The model under review builds one solid part; all positions refer to its coordinate system, in mm. Round coordinates to 2 decimals unless told otherwise and drop trailing zeros. Order: outer loops, then holes, each group sorted by start corner. A loop starts at its lowest first (then second) coordinate and runs counter-clockwise, first axis right, second up.
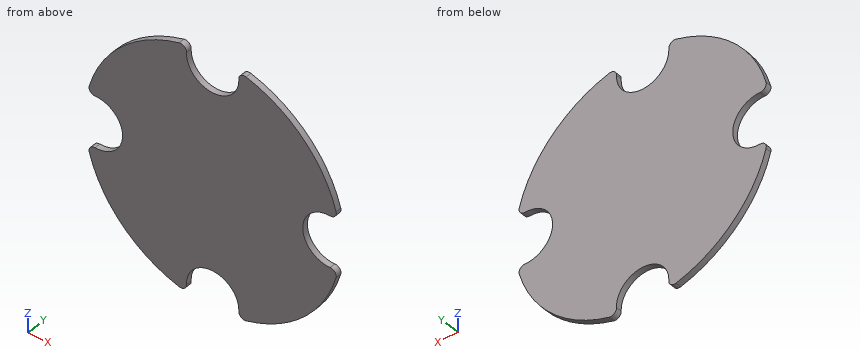
Autodesk Fusion 360 part; units mm, degrees
sketch "Sketch1" plane through (0, 0, 0) normal (0, 1, 0) x (1, 0, 0)
  circle A0 centre (0, 0) radius 10 construction
  circle A1 centre (10, 0) radius 2.25
  circle A2 centre (0, 10) radius 2.25
  circle A3 centre (-10, 0) radius 2.25
  circle A4 centre (0, -10) radius 2.25
  circle A5 centre (0, 0) radius 11
  dimension "d1" = 20
  dimension "d2" = 4.5
  dimension "d4" = 360
  dimension "d5" = 22
extrude "Extrude1" add sketch "Sketch1" along normal blind 0.5 contours A1 A2 A3 A4 A5
fillet "Fillet1" radius 0.5 8 edges at (-2.1042, 0.25, 10.7969) (2.1042, 0.25, 10.7969) (-10.7969, 0.25, 2.1042) (-10.7969, 0.25, -2.1042) (-2.1042, 0.25, -10.7969) (2.1042, 0.25, -10.7969) (10.7969, 0.25, -2.1042) (10.7969, 0.25, 2.1042)
(1) We need section C-C (x = 0). Give the boundary of the cut face in (y, z).
(2) We need section B-B (x = -8). Give the boundary of the cut face in (y, z), and give its area (3 significant figures).
(3) To check wall thickness, follow L1, parallel to Z at x = -8.75, y = 0.45; L2, parallel to Z at x = -8.5, y = 0.15. State the ranges of each line that lie inside material, in increasing order.
(4) We need section A-A (x = 9.25). Give the boundary of the cut face in (y, z), and give its area (3 significant figures).
(5) We need section D-D (z = -6.5). Give the boundary of the cut face in (x, y).
Verdict:
1. outline: (0, -7.75) - (0.5, -7.75) - (0.5, 7.75) - (0, 7.75) - close
2. outline: (0, -7.55) - (0.5, -7.55) - (0.5, -1.03) - (0, -1.03) - close; (0, 1.03) - (0.5, 1.03) - (0.5, 7.55) - (0, 7.55) - close
2. area: 6.52 mm2
3. L1: z = -6.67 to -1.87, 1.87 to 6.67
3. L2: z = -6.98 to -1.68, 1.68 to 6.98
4. outline: (0, -5.95) - (0.5, -5.95) - (0.5, -2.12) - (0, -2.12) - close; (0, 2.12) - (0.5, 2.12) - (0.5, 5.95) - (0, 5.95) - close
4. area: 3.83 mm2
5. outline: (-8.87, 0) - (8.87, 0) - (8.87, 0.5) - (-8.87, 0.5) - close
